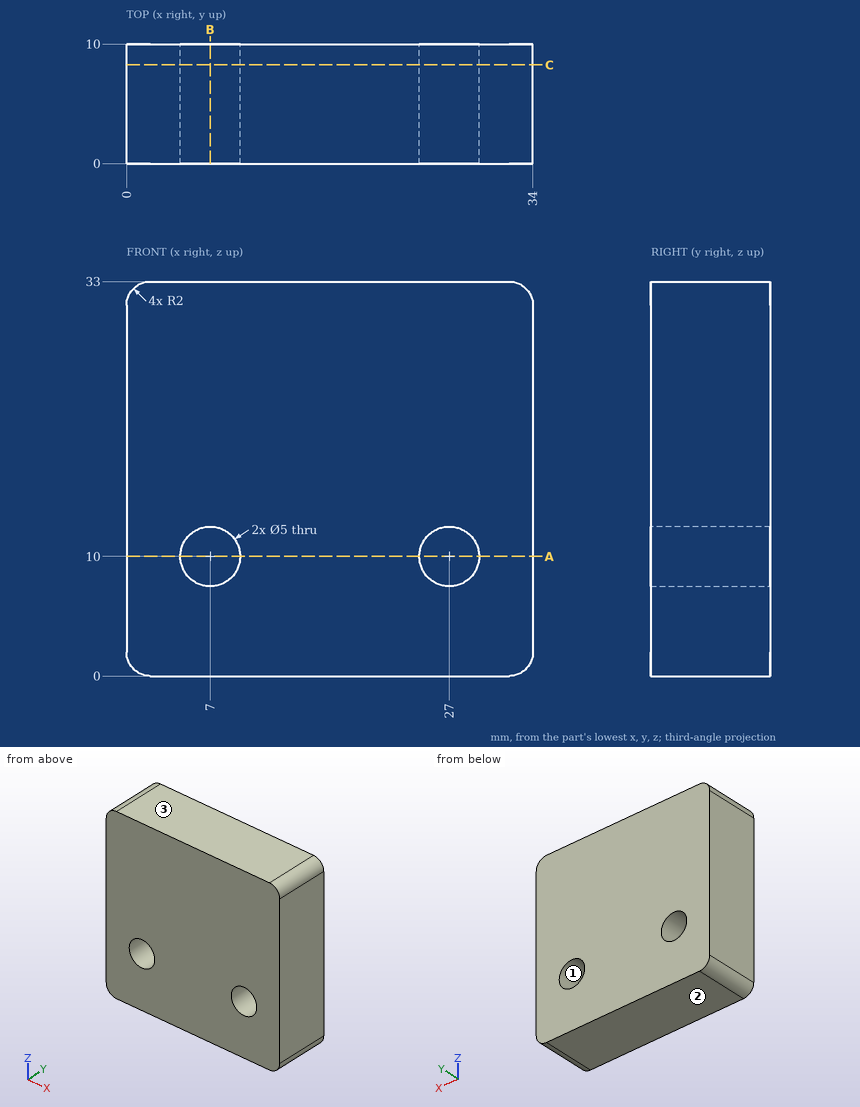
Geometry: see drawing. Coordinates: mm, zero at the bounding-box minimum. Give positions to 0.01 mm unless a question says otherwise; leave off trailing zeros. Loops run counter-clockwise (first coordinate to the right, second up) from the corner with the lowest first, then second, coordinate; pieces in that order, holes last. Notation, with made-up numbers: (62, 6.5) - (117, 6.5) arc R24 cw to (117, 18.5) - close; hole circle Ø6 at (56.25, -36.5). An arc over 180 degrees is marked (long way). Use CSV: the item, a comma, the result in double quotes. Start each with the question number.
Item 1: Section B-B on x = 7. Return loops of the section in (y, z), then the cut area to 3 significant figures.
Item 2: Line query: line 1 (X direction, y = 2, z = 10); line 2 (X direction, y = 4.25, z = 8.5); line 3 (Z direction, x = 5.5, y = 5). Output: solid intervals per line, ascending.
Item 3: Contact query for flat-ended pins moving along their axis: P1, Ø8, axis at x = 4, z = 29, coming from the -Y side; P2, Ø4, axis at x = 27, z = 10, coming from the -Y side. Output: stop coordinate, or through.
Item 4: Section A-A on z = 10. Return loops of the section in (x, y), then the cut area to 3 significant figures.
Item 5: Mould query, pull axis Z, two halves, no side actions, for the marked faces 1, 2 and 3. Classes: pulls with the +Z half, pulls with the -Z half, needs draft (parallel to the pull), parting line crosses it, or undercut.
Item 6: Section C-C on y = 8.25. Return loops of the section in (x, z).
Ans:
1,outline,"(0, 0) - (10, 0) - (10, 7.5) - (0, 7.5) - close; (0, 12.5) - (10, 12.5) - (10, 33) - (0, 33) - close"
1,area,"280 mm2"
2,line 1,"x = 0 to 4.5, 9.5 to 24.5, 29.5 to 34"
2,line 2,"x = 0 to 5, 9 to 25, 29 to 34"
2,line 3,"z = 0 to 8, 12 to 33"
3,P1,"stops at y = 0"
3,P2,"passes through"
4,outline,"(0, 0) - (4.5, 0) - (4.5, 10) - (0, 10) - close; (9.5, 0) - (24.5, 0) - (24.5, 10) - (9.5, 10) - close; (29.5, 0) - (34, 0) - (34, 10) - (29.5, 10) - close"
4,area,"240 mm2"
5,face 1,"undercut"
5,face 2,"pulls with the -Z half"
5,face 3,"pulls with the +Z half"
6,outline,"(0, 2) arc R2 ccw to (2, 0) - (32, 0) arc R2 ccw to (34, 2) - (34, 31) arc R2 ccw to (32, 33) - (2, 33) arc R2 ccw to (0, 31) - close; hole circle Ø5 at (7, 10); hole circle Ø5 at (27, 10)"
